Geometry check sheet. Reference: the model listing, model coordinates, mm. A direction names the side the tool comes from. Round coordinates to 2 decimals unless told otherwise and drop trailing zeros. Loops run counter-clockwise (first coordinate to the right, second up) from the corner with the lowest first, then second, coordinate; pieces in that order, holes last. Notation, with made-up numbers: (77.5, -33) -> (131.5, -33) arc R32 ccw to (131.5, -3) -> close; hole circle Ø5 at (61, 64). An arc over 180 degrees is marked (long way). Use a Markdown table: item, result. Add a question column.
Q1. Sectioned sample at B-B, the plane z = 5.5. Enter the section's corners in (x, y), then the cut area to 3 significant figures.
Q2. Sectioned sample at D-D, the plane y = 432.5. Enter the section's corners in (x, z), then the cut area to 3 significant figures.
Q3. Release check for a two-part mould opening along X. For faces 6 (the face through (-2, 421.899, 5)), 7 (the face through (13.531, 483, 5)), 8 (the face through (8, 482, 9.956)) record: released by +X, released by -X, zero draft, split by the parting line, or undercut.
Q4. Gauge pin test, flat ends, axial feed: P1, Ø3, axis at y = 485, z = 6.5, coming from the +X side; P2, Ø3, axis at x = -9.5, y = 480.5, coming from the +Z side; P3, Ø3, axis at x = -19, y = 437, coming from the -Z side. Record the tip position at first contact, or that the pin passes through.
Q5. Sectioned sample at C-C, the plane x = -12. Enter the section's corners in (y, z), then the cut area to 3 significant figures.
Q6. Sectioned sample at A-A, the plane x = -4.5. Enter the section's corners in (y, z), then the cut area to 3 significant figures.
Q7. Set-up check for faces 1 (the face through (17, 433.899, -4)), 2 (the face through (6.531, 465, -3)), 3 (the face through (-16.969, 437, 5)), 4 (the face through (-12, 482, -0.044)), 5 (the face through (-6.469, 483, 5)): record each of +Z, -Z, +X, -X, +Y, -Y from which the full face is reachable in a straight line by a thin tool's end or side.
Q8. Material ranges on L1, parallel to X at y = 439.5, z = -2; L2, parallel to Y at x = 1, z = 9.5; L3, parallel to X at y = 480.5, z = 9, recorded low to high.
```python
from build123d import *

# Parameters (mm, degrees)
SKETCH1_W           = 50
SKETCH1_H           = 40
BOSS_EXTRUDE1_DEPTH = 10
SKETCH5_W           = 6
SKETCH5_H           = 5
BOSS_EXTRUDE3_DEPTH = 10
SKETCH6_R           = 2
CUT_EXTRUDE1_DEPTH  = 20
SKETCH8_W           = 10
SKETCH8_H           = 40
CUT_EXTRUDE2_DEPTH  = 25
SKETCH9_W           = 10
SKETCH9_H           = 6
SKETCH9_R           = 1.930897171
BOSS_EXTRUDE4_DEPTH = 5
SKETCH10_W          = 10
SKETCH10_H          = 5
CUT_EXTRUDE3_DEPTH  = 15
SKETCH11_W          = 5
SKETCH11_H          = 5
BOSS_EXTRUDE5_DEPTH = 10
SKETCH12_R          = 1.5
CUT_EXTRUDE4_DEPTH  = 10
SKETCH13_W          = 6
SKETCH13_H          = 5
CUT_EXTRUDE5_DEPTH  = 10
SKETCH15_W          = 5
SKETCH15_H          = 5
BOSS_EXTRUDE7_DEPTH = 10
SKETCH18_W          = 5
SKETCH18_H          = 5
CUT_EXTRUDE7_DEPTH  = 10
SKETCH19_R          = 1.25
CUT_EXTRUDE8_DEPTH  = 43
CUT_EXTRUDE9_DEPTH  = 20
SKETCH21_W          = 15.5
SKETCH21_H          = 15.5
CUT_EXTRUDE10_DEPTH = 30
SKETCH22_W          = 8
SKETCH22_H          = 12.25
CUT_EXTRUDE11_DEPTH = 2
SCALE2_SCALE        = 2
CUT_EXTRUDE12_DEPTH = 30
SKETCH24_W          = 44
SKETCH24_H          = 7
CUT_EXTRUDE13_DEPTH = 3


with BuildPart() as part:
    # Sketch1 → Boss-Extrude1 (new body)
    with BuildSketch(Plane(origin=(669.84184187, 0, 0), x_dir=(1, 0, 0), z_dir=(0, 0, 1))):
        with Locations((-671.310344828, 437.637931034)):
            Rectangle(SKETCH1_W, SKETCH1_H)
    boss_extrude1 = extrude(amount=BOSS_EXTRUDE1_DEPTH)

    # Sketch5 → Boss-Extrude3 (add)
    with BuildSketch(Plane(origin=(23.531497042, 0, 0), x_dir=(0, 0, -1), z_dir=(1, 0, 0))):
        with Locations((-5, 442.637931034)):
            Rectangle(SKETCH5_W, SKETCH5_H)
        with Locations((-5, 432.637931034)):
            Rectangle(SKETCH5_W, SKETCH5_H)
    extrude(amount=BOSS_EXTRUDE3_DEPTH)

    # Sketch6 → Cut-Extrude1 (cut)
    with BuildSketch(Plane(origin=(669.84184187, 445.137931034, 0), x_dir=(1, 0, 0), z_dir=(0, 1, 0))):
        with Locations(Location((-641.310344828, -5, 0), (0, 0, 180))):
            Circle(SKETCH6_R)
    extrude(amount=-CUT_EXTRUDE1_DEPTH, mode=Mode.SUBTRACT)

    # Sketch8 → Cut-Extrude2 (cut)
    with BuildSketch(Plane.ZY.offset(26.468502958)):
        with Locations((5, 437.637931034)):
            Rectangle(SKETCH8_W, SKETCH8_H)
    extrude(amount=-CUT_EXTRUDE2_DEPTH, mode=Mode.SUBTRACT)

    # Sketch9 → Boss-Extrude4 (add)
    with BuildSketch(Plane(origin=(0, 435.137931034, 0), x_dir=(1, 0, 0), z_dir=(0, 1, 0))):
        with Locations((28.531497042, -5)):
            Rectangle(SKETCH9_W, SKETCH9_H)
        with Locations(Location((28.531497042, -5, 0), (0, 0, 180))):
            Circle(SKETCH9_R, mode=Mode.SUBTRACT)
    extrude(amount=BOSS_EXTRUDE4_DEPTH)

    # Sketch10 → Cut-Extrude3 (cut)
    with BuildSketch(Plane.XY.offset(8)):
        with Locations((28.531497042, 432.637931034)):
            Rectangle(SKETCH10_W, SKETCH10_H)
        with Locations((28.531497042, 442.637931034)):
            Rectangle(SKETCH10_W, SKETCH10_H)
    extrude(amount=-CUT_EXTRUDE3_DEPTH, mode=Mode.SUBTRACT)

    # Mirror1: Boss-Extrude1 across plane
    add(boss_extrude1.mirror(Plane(origin=(-1.468502958, 0, 0), x_dir=(0, 0, 1), z_dir=(1, 0, 0))))

    # Sketch11 → Boss-Extrude5 (add)
    with BuildSketch(Plane(origin=(0, 457.637931034, 0), x_dir=(1, 0, 0), z_dir=(0, 1, 0))):
        with Locations((-1.468502958, -5)):
            Rectangle(SKETCH11_W, SKETCH11_H)
    extrude(amount=BOSS_EXTRUDE5_DEPTH)

    # Sketch12 → Cut-Extrude4 (cut)
    with BuildSketch(Plane(origin=(1.031497042, 0, 0), x_dir=(0, 0, -1), z_dir=(1, 0, 0))):
        with Locations((-5, 462.637931034)):
            Circle(SKETCH12_R)
    extrude(amount=-CUT_EXTRUDE4_DEPTH, mode=Mode.SUBTRACT)

    # Sketch13 → Cut-Extrude5 (cut)
    with BuildSketch(Plane(origin=(33.531497042, 0, 0), x_dir=(0, 0, -1), z_dir=(1, 0, 0))):
        with Locations((-5, 437.637931034)):
            Rectangle(SKETCH13_W, SKETCH13_H)
    extrude(amount=-CUT_EXTRUDE5_DEPTH, mode=Mode.SUBTRACT)

    # Sketch15 → Boss-Extrude7 (add)
    with BuildSketch(Plane(origin=(0, 457.637931034, 0), x_dir=(1, 0, 0), z_dir=(0, 1, 0))):
        with Locations((-6.468502958, -5)):
            Rectangle(SKETCH15_W, SKETCH15_H)
        with Locations((3.531497042, -5)):
            Rectangle(SKETCH15_W, SKETCH15_H)
    extrude(amount=BOSS_EXTRUDE7_DEPTH)

    # Sketch18 → Cut-Extrude7 (cut)
    with BuildSketch(Plane(origin=(0, 467.637931034, 0), x_dir=(1, 0, 0), z_dir=(0, 1, 0))):
        with Locations((-1.468502958, -5)):
            Rectangle(SKETCH18_W, SKETCH18_H)
    extrude(amount=-CUT_EXTRUDE7_DEPTH, mode=Mode.SUBTRACT)

    # Sketch19 → Cut-Extrude8 (cut)
    with BuildSketch(Plane.ZY.offset(8.968502958)):
        with Locations((5, 462.637931034)):
            Circle(SKETCH19_R)
    extrude(amount=-CUT_EXTRUDE8_DEPTH, mode=Mode.SUBTRACT)

    # Sketch20 → Cut-Extrude9 (cut)
    with BuildSketch(Plane(origin=(6.031497042, 0, 0), x_dir=(0, 0, -1), z_dir=(1, 0, 0))):
        with BuildLine():
            Line((-7.5, 467.637931034), (-7.5, 462.637931034))
            ThreePointArc((-7.5, 462.637931034), (-5, 465.137931034), (-2.5, 462.637931034))
            Line((-2.5, 462.637931034), (-2.5, 467.637931034))
            Line((-2.5, 467.637931034), (-7.5, 467.637931034))
        make_face()
    extrude(amount=-CUT_EXTRUDE9_DEPTH, mode=Mode.SUBTRACT)

    # Sketch21 → Cut-Extrude10 (cut)
    with BuildSketch(Plane.XY.offset(10)):
        with Locations((-1.468502958, 437.637931034)):
            Rectangle(SKETCH21_W, SKETCH21_H)
    extrude(amount=-CUT_EXTRUDE10_DEPTH, mode=Mode.SUBTRACT)

    # Sketch22 → Cut-Extrude11 (cut)
    with BuildSketch(Plane(origin=(0, 0, 0), x_dir=(-1, 0, 0), z_dir=(0, 0, -1))):
        with Locations((1.468502958, 451.512931034)):
            Rectangle(SKETCH22_W, SKETCH22_H)
    extrude(amount=-CUT_EXTRUDE11_DEPTH, mode=Mode.SUBTRACT)


with BuildPart() as part_1:
    # Scale2: scaled about (-1.468502958, 437.877293221, 5.044292315)
    add(part.part.scale(SCALE2_SCALE).moved(Location((1.468502958, -437.877293221, -5.044292315))))

    # Sketch23 → Cut-Extrude12 (cut)
    with BuildSketch(Plane(origin=(0, 0, -5.044292315), x_dir=(-1, 0, 0), z_dir=(0, 0, -1))):
        Polygon((26.968502958, 495.287404552), (26.968502958, 477.398568848), (51.468502958, 477.398568848), (51.468502958, 397.398568848), (-48.531497042, 397.398568848), (-48.531497042, 477.398568848), (-24.031497042, 477.398568848), (-24.031497042, 495.287404552), (-71.530370383, 495.287404552), (-71.530370383, 371.111775085), (85.960671869, 371.111775085), (85.960671869, 495.287404552), align=None)
        Polygon((51.468502958, 477.398568848), (26.968502958, 477.398568848), (26.968502958, 410.898568848), (-24.031497042, 410.898568848), (-24.031497042, 477.398568848), (-48.531497042, 477.398568848), (-48.531497042, 397.398568848), (51.468502958, 397.398568848), align=None)
    extrude(amount=-CUT_EXTRUDE12_DEPTH, mode=Mode.SUBTRACT)

    # Sketch24 → Cut-Extrude13 (cut)
    with BuildSketch(Plane(origin=(0, 0, -5.044292315), x_dir=(-1, 0, 0), z_dir=(0, 0, -1))):
        with Locations((1.468502958, 437.398568848)):
            Rectangle(SKETCH24_W, SKETCH24_H)
    extrude(amount=-CUT_EXTRUDE13_DEPTH, mode=Mode.SUBTRACT)


solid = part_1.part
```
Values:
| question | item | result |
|---|---|---|
| 1 | outline | (-26.97, 410.9) -> (24.03, 410.9) -> (24.03, 477.4) -> (13.53, 477.4) -> (13.53, 484.96) -> (3.53, 484.96) -> (3.53, 477.4) -> (-6.47, 477.4) -> (-6.47, 484.96) -> (-16.47, 484.96) -> (-16.47, 477.4) -> (-26.97, 477.4) -> close; (-16.47, 489.84) -> (-6.47, 489.84) -> (-6.47, 492.37) -> (-16.47, 492.37) -> close; (3.53, 489.84) -> (13.53, 489.84) -> (13.53, 492.37) -> (3.53, 492.37) -> close; hole (-16.97, 421.9) -> (14.03, 421.9) -> (14.03, 452.9) -> (-16.97, 452.9) -> close |
| 1 | area | 2,630 mm^2 |
| 2 | outline | (-26.97, -5.04) -> (-16.97, -5.04) -> (-16.97, 14.96) -> (-26.97, 14.96) -> close; (14.03, -5.04) -> (24.03, -5.04) -> (24.03, 14.96) -> (14.03, 14.96) -> close |
| 2 | area | 400 mm^2 |
| 3 | face 6 | undercut |
| 3 | face 7 | released by +X |
| 3 | face 8 | zero draft |
| 4 | P1 | x = 13.53 |
| 4 | P2 | z = 9.96 |
| 4 | P3 | z = -2.04 |
| 5 | outline | (410.9, -5.04) -> (421.9, -5.04) -> (421.9, 14.96) -> (410.9, 14.96) -> close; (452.9, -5.04) -> (477.4, -5.04) -> (477.4, -0.04) -> (487.4, -0.04) arc R5 ccw to (487.4, 9.96) -> (477.4, 9.96) -> (477.4, 14.96) -> (452.9, 14.96) -> close; hole circle Ø5 at (487.4, 4.96) |
| 5 | area | 830 mm^2 |
| 6 | outline | (410.9, -5.04) -> (421.9, -5.04) -> (421.9, 14.96) -> (410.9, 14.96) -> close; (452.9, -1.04) -> (477.4, -1.04) -> (477.4, 14.96) -> (452.9, 14.96) -> close |
| 6 | area | 612 mm^2 |
| 7 | face 1 | -Z |
| 7 | face 2 | -Z, +Y |
| 7 | face 3 | +Z, -Z |
| 7 | face 4 | -Z, +X, -X, +Y |
| 7 | face 5 | +Z, -Z, +Y |
| 8 | L1 | -26.97 to -16.97, 14.03 to 24.03 |
| 8 | L2 | 410.9 to 421.9, 452.9 to 477.4 |
| 8 | L3 | -16.47 to -6.47, 3.53 to 13.53 |
